Can you work these out from the model? Positions are in its coordinate system, mm. A direction names the side the tool comes from. Coordinates: 2 decimals unless noted, no trailing zeros. Loops run counter-clockwise (first coordinate to the right, second up) from the corner with the lowest first, then second, coordinate; pieces in that order, holes last. Notation, with made-up numbers: M -25.5,72.5 L 3.5,72.5 A10 cw 3.5,84.5 Z; hole C -35,-4 d4. An arc over 180 degrees is marked long. Answer as a JSON object with one key per item and string values. Group by question number.
Item 1: If I drill on line 1 (X direction, y = 10, z = -27.94) (3 decimals); line 2 (Y direction, x = -2, z = -29.5) (3 decimals); line 3 (Z direction, x = -38, y = 6.75), over which ranges is the centre line in solid material (lowest first)?
Item 2: Suppose I cut it at B-B (x = -14). Write out the boundary of the cut face in (y, z) (3 decimals), then the cut area to 3 significant figures.
Item 3: Suppose I cut it at C-C (z = -2). Write out the boundary of the cut face in (x, y) (3 decimals), then the cut area to 3 significant figures.
Item 4: Suppose I cut it at A-A (y = 8.5). Write out the boundary of the cut face in (x, z) (3 decimals), then the cut area to 3 significant figures.
Item 5: Which directions (+Z, -Z, +X, -X, +Y, -Y) give clear straight access to the entire face, cutting with the end or side of a thin tool? Please do faces 1 (the cylindrical face through (-42.977, 9.436, 32.046)), 2 (the flat face through (45, 3.175, -31)), 3 (the flat face through (-1, 2, 32.385)).
Item 6: I'm going to push flat-ended pins straight in: pin 1 Ø19.5 at (x, z) = (-8.5, 14.5) entering from +Y (3 decimals); pin 2 Ø8 at (y, z) = (11, -5.5) entering from -X. Where does each tip first touch, or does it pass through?
Item 7: We'd pull the mould along X, two halves only. Please class faces 4 (the cylindrical face through (44.956, 1.61, -31.661)), 5 (the cylindrical face through (-44.996, 1.61, 31.621)), 6 (the cylindrical face through (40.24, 8.05, -29.29)), 7 (the flat face through (41, 15.875, -30)): +X half, -X half, draft (parallel to the pull), parting line (faces both ways), or undercut.
```python
from build123d import *

# Parameters (mm, degrees)
SKETCH1_W           = 91.44
SKETCH1_H           = 64.77
BOSS_EXTRUDE1_DEPTH = 3.175
SKETCH2_R           = 4.445
BOSS_EXTRUDE2_DEPTH = 12.7
SKETCH3_R           = 1.6999966
CUT_EXTRUDE1_DEPTH  = 59.233343112
FILLET1_R           = 2.54


with BuildPart() as part:
    # Sketch1 → Boss-Extrude1 (new body)
    with BuildSketch(Plane(origin=(0, 0, 0), x_dir=(1, 0, 0), z_dir=(0, 1, 0))):
        Rectangle(SKETCH1_W, SKETCH1_H)
    extrude(amount=BOSS_EXTRUDE1_DEPTH)

    # Sketch2 → Boss-Extrude2 (add)
    with BuildSketch(Plane(origin=(0, 3.175, 0), x_dir=(1, 0, 0), z_dir=(0, 1, 0))):
        with Locations(Location((-41.275, 27.94, 0), (0, 0, 90))):
            Circle(SKETCH2_R)
        with Locations(Location((41.275, 27.94, 0), (0, 0, 90))):
            Circle(SKETCH2_R)
        with Locations(Location((41.275, -27.94, 0), (0, 0, 270))):
            Circle(SKETCH2_R)
        with Locations(Location((-41.275, -27.94, 0), (0, 0, 270))):
            Circle(SKETCH2_R)
    extrude(amount=BOSS_EXTRUDE2_DEPTH)

    # Sketch3 → Cut-Extrude1 (cut, through all)
    with BuildSketch(Plane(origin=(0, 15.875, 0), x_dir=(1, 0, 0), z_dir=(0, 1, 0))):
        with Locations(Location((-41.275, 27.94, 0), (0, 0, 270))):
            Circle(SKETCH3_R)
        with Locations(Location((41.275, 27.94, 0), (0, 0, 270))):
            Circle(SKETCH3_R)
        with Locations(Location((41.275, -27.94, 0), (0, 0, 270))):
            Circle(SKETCH3_R)
        with Locations(Location((-41.275, -27.94, 0), (0, 0, 270))):
            Circle(SKETCH3_R)
    extrude(amount=-CUT_EXTRUDE1_DEPTH, mode=Mode.SUBTRACT)

    # Fillet1
    fillet1_edges = [part.edges().sort_by_distance(p)[0] for p in [
        (45.72, 1.5875, 32.385),
        (-45.72, 1.5875, 32.385),
        (-45.72, 1.5875, -32.385),
        (45.72, 1.5875, -32.385),
    ]]
    fillet(fillet1_edges, radius=FILLET1_R)


solid = part.part
```
From the geometry:
{
 "1": {"line 1": "-45.72 to -42.975, -39.575 to -36.83, 36.83 to 39.575, 42.975 to 45.72", "line 2": "0 to 3.175", "line 3": "-30.95 to -24.93, 24.93 to 30.95"},
 "2": {"outline": "M 0,-32.385 L 3.175,-32.385 L 3.175,32.385 L 0,32.385 Z", "area": "206 mm2"},
 "3": {"outline": "M -45.72,0 L 45.72,0 L 45.72,3.175 L -45.72,3.175 Z", "area": "290 mm2"},
 "4": {"outline": "C -41.275,-27.94 d8.89; C -41.275,27.94 d8.89; C 41.275,-27.94 d8.89; C 41.275,27.94 d8.89; hole C -41.275,-27.94 d3.4; hole C -41.275,27.94 d3.4; hole C 41.275,-27.94 d3.4; hole C 41.275,27.94 d3.4", "area": "212 mm2"},
 "5": {"face 1": "+Y", "face 2": "-Z, +X, +Y", "face 3": "+Z, +X, -X, +Y, -Y"},
 "6": {"pin 1": "y = 3.175", "pin 2": "through"},
 "7": {"face 4": "+X half", "face 5": "-X half", "face 6": "undercut", "face 7": "draft"}
}
